For this review, take the finished solid that the model builds, in its own axes (mm). A direction names the side the tool comes from. Round coordinates to 2 decimals unless told otherwise and drop trailing zeros. Loops run counter-clockwise (first coordinate to the right, second up) from the corner with the lowest first, then second, coordinate; pieces in that order, holes last. Notation, with made-up numbers: M 62.5,-7 L 116.5,-7 A19 cw 116.5,11 Z; hole C 67.25,2.25 d2. An arc over 180 degrees is marked long. One line per question, with ' | ' between items. Start each with the question number.
1) We need section C-C (x = -8). Give the boundary of the cut face in (y, z), and give its area (3 significant figures).
2) Mouldability with a two-part tool opening along Z and no side actions: class faces 1 (the face through (-71.05, -17.27, -73.83)), 2 (the face through (-44, 8, -72.784)), 3 (the face through (-44, 15.7, -9)) as pulls with the +Z half, pulls with the -Z half, needs draft (parallel to the pull), parting line crosses it, or undercut.
3) For pin 1 Ø17 at (x, z) = (-32.55, -73.48) entering from -Y; pin 2 Ø6.5 at (x, z) = (-32.55, -73.48) entering from +Y; pin 3 Ø3 at (x, z) = (-74, -68.5) entering from -Y; pin 4 Ø17.5 at (y, z) = (6, -40) entering from -X, all flat-tipped, find the tip position at first contact; note any pin that passes through.
4) For faces 4 (the face through (-44, 21, -49.384)), 5 (the face through (-44, -17, -57.784)), 6 (the face through (-76.39, -6.03, -56.04)), 7 (the face through (-12, 21, -27.09)), list the 3-axis set-ups (+Z, -Z, +X, -X, +Y, -Y) from which the entire face can be reached by the end or side of a thin tool; tool diameter is ignored.
5) For probe 1 along X at (y, z) = (7, -54); probe 2 along X at (y, z) = (17, -56.5); probe 3 along Z at (x, y) = (-67.5, -2.5), list the stretches that pass through material, from the lowest coordinate up. Write a range as from..to.
6) We need section B-B (z = -39). Give the boundary of the cut face in (x, y).
7) We need section A-A (y = -18). State how many separate pieces and enclosed holes the cut face has, and give its area (3 significant figures).
```python
from build123d import *

# Parameters (mm, degrees)
SZKIC1_W                     = 44
SZKIC1_H                     = 78
DODANIE_WYCI_GNI_CIE1_DEPTH  = 15.7
SZKIC2_W                     = 54.82
SZKIC2_H                     = 26
DODANIE_WYCI_GNI_CIE2_DEPTH  = 10
DODANIE_WYCI_GNI_CIE3_DEPTH  = 1
SZKIC6_R                     = 10.4
SZKIC6_R_2                   = 4
DODANIE_WYCI_GNI_CIE4_DEPTH  = 33
SZKIC7_R                     = 10.5
DODANIE_WYCI_GNI_CIE5_DEPTH  = 33
DODANIE_WYCI_GNI_CIE6_DEPTH  = 33
DODANIE_WYCI_GNI_CIE22_DEPTH = 10
SZKIC15_R                    = 3
DODANIE_WYCI_GNI_CIE23_DEPTH = 6.525


with BuildPart() as part:
    # Szkic1 → Dodanie-wyciągnięcie1 (new body)
    with BuildSketch(Plane(origin=(0, 0, 0), x_dir=(1, 0, 0), z_dir=(0, 1, 0))):
        with Locations((-44.05199022, 33.7842123)):
            Rectangle(SZKIC1_W, SZKIC1_H)
    extrude(amount=DODANIE_WYCI_GNI_CIE1_DEPTH)

    # Szkic2 → Dodanie-wyciągnięcie2 (add)
    with BuildSketch(Plane(origin=(0, 15.7, 0), x_dir=(1, 0, 0), z_dir=(0, 1, 0))):
        with Locations((-44.05199022, 36.3842123)):
            Rectangle(SZKIC2_W, SZKIC2_H)
    extrude(amount=DODANIE_WYCI_GNI_CIE2_DEPTH)

    # Szkic3 → Dodanie-wyciągnięcie3 (add)
    with BuildSketch(Plane.XZ):
        with BuildLine():
            Line((-32.55199022, -89.3842123), (-55.55199022, -89.3842123))
            ThreePointArc((-55.55199022, -89.3842123), (-71.45199022, -73.4842123), (-55.55199022, -57.5842123))
            Line((-55.55199022, -57.5842123), (-32.55199022, -57.5842123))
            ThreePointArc((-32.55199022, -57.5842123), (-16.65199022, -73.4842123), (-32.55199022, -89.3842123))
        make_face()
    extrude(amount=DODANIE_WYCI_GNI_CIE3_DEPTH)

    # Szkic6 → Dodanie-wyciągnięcie4 (add)
    with BuildSketch(Plane(origin=(0, -1, 0), x_dir=(-1, 0, 0), z_dir=(0, -1, 0))):
        with Locations((32.55199022, 73.4842123)):
            Circle(SZKIC6_R)
        with Locations((32.55199022, 73.4842123)):
            Circle(SZKIC6_R_2, mode=Mode.SUBTRACT)
        with Locations((55.55199022, 73.4842123)):
            Circle(SZKIC6_R)
        with Locations((55.55199022, 73.4842123)):
            Circle(SZKIC6_R_2, mode=Mode.SUBTRACT)
    extrude(amount=DODANIE_WYCI_GNI_CIE4_DEPTH)

    # Szkic7 → Dodanie-wyciągnięcie5 (add)
    with BuildSketch(Plane(origin=(0, -1, 0), x_dir=(-1, 0, 0), z_dir=(0, -1, 0))):
        with BuildLine():
            Line((55.55199022, 57.9842123), (32.55199022, 57.9842123))
            ThreePointArc((32.55199022, 57.9842123), (17.05199022, 73.4842123), (32.55199022, 88.9842123))
            Line((32.55199022, 88.9842123), (55.55199022, 88.9842123))
            ThreePointArc((55.55199022, 88.9842123), (71.05199022, 73.4842123), (55.55199022, 57.9842123))
        make_face()
        with Locations((55.55199022, 73.4842123)):
            Circle(SZKIC7_R, mode=Mode.SUBTRACT)
        with Locations((32.55199022, 73.4842123)):
            Circle(SZKIC7_R, mode=Mode.SUBTRACT)
    extrude(amount=DODANIE_WYCI_GNI_CIE5_DEPTH)

    # Szkic8 → Dodanie-wyciągnięcie6 (add)
    with BuildSketch(Plane(origin=(0, -1, 0), x_dir=(-1, 0, 0), z_dir=(0, -1, 0))):
        with BuildLine():
            Line((32.55199022, 57.5842123), (55.55199022, 57.5842123))
            ThreePointArc((55.55199022, 57.5842123), (71.45199022, 73.4842123), (55.55199022, 89.3842123))
            Line((55.55199022, 89.3842123), (32.55199022, 89.3842123))
            ThreePointArc((32.55199022, 89.3842123), (16.65199022, 73.4842123), (32.55199022, 57.5842123))
        make_face()
        with BuildLine():
            Line((55.55199022, 57.7842123), (32.55199022, 57.7842123))
            ThreePointArc((32.55199022, 57.7842123), (16.85199022, 73.4842123), (32.55199022, 89.1842123))
            Line((32.55199022, 89.1842123), (55.55199022, 89.1842123))
            ThreePointArc((55.55199022, 89.1842123), (71.25199022, 73.4842123), (55.55199022, 57.7842123))
        make_face(mode=Mode.SUBTRACT)
    extrude(amount=DODANIE_WYCI_GNI_CIE6_DEPTH)

    # Szkic13 → Dodanie-wyciągnięcie22 (add)
    with BuildSketch(Plane(origin=(-16.64199022, 0, 0), x_dir=(0, 0, -1), z_dir=(1, 0, 0))):
        with BuildLine():
            Line((63.214194972, -27.158978782), (48.662895357, 15.7))
            Line((48.662895357, 15.7), (27.090339285, 15.7))
            Line((27.090339285, 15.7), (27.090339285, 25.7))
            Line((27.090339285, 25.7), (59.347416053, 25.7))
            Line((59.347416053, 25.7), (72.7842123, 8.659604885))
            Line((72.7842123, 8.659604885), (77.184359271, 12.129235601))
            Line((77.184359271, 12.129235601), (105.9842123, -20.239479664))
            ThreePointArc((105.9842123, -20.239479664), (86.046845732, -32.647229139), (63.214194972, -27.158978782))
        make_face()
    dodanie_wyci_gni_cie22 = extrude(amount=DODANIE_WYCI_GNI_CIE22_DEPTH)

    # Lustro2: Dodanie-wyciągnięcie22 across plane
    add(dodanie_wyci_gni_cie22.mirror(Plane(origin=(-44.05199022, 0, 0), x_dir=(0, 0, 1), z_dir=(1, 0, 0))))

    # Szkic15 → Dodanie-wyciągnięcie23 (add)
    with BuildSketch(Plane(origin=(-6.64199022, 0, 0), x_dir=(0, 0, -1), z_dir=(1, 0, 0))):
        with Locations((98.903450656, -19.74322341)):
            Circle(SZKIC15_R)
    dodanie_wyci_gni_cie23 = extrude(amount=DODANIE_WYCI_GNI_CIE23_DEPTH)

    # Lustro3: Dodanie-wyciągnięcie23 across plane
    add(dodanie_wyci_gni_cie23.mirror(Plane(origin=(-44.05199022, 0, 0), x_dir=(0, 0, 1), z_dir=(1, 0, 0))))


solid = part.part
```
Answers below:
1) outline: M -27.16,-63.21 A30.42 ccw -20.24,-105.98 L 12.13,-77.18 L 8.66,-72.78 L 25.7,-59.35 L 25.7,-27.09 L 15.7,-27.09 L 15.7,-48.66 Z | area: 2,020 mm^2
2) face 1: undercut | face 2: pulls with the -Z half | face 3: needs draft
3) pin 1: y = -34 | pin 2: y = 15.7 | pin 3: y = -30.91 | pin 4: x = -66.05
4) face 4: -Z, +Y | face 5: -Y | face 6: +Z, -X, -Y | face 7: +Z, +X, +Y, -Y
5) probe 1: -81.46..-71.46, -66.05..-22.05, -16.64..-6.64 | probe 2: -81.46..-71.46, -16.64..-6.64 | probe 3: -83.97..-83.67, -83.36..-63.61, -63.3..-62.99
6) outline: M -81.46,15.7 L -66.05,15.7 L -66.05,0 L -22.05,0 L -22.05,15.7 L -6.64,15.7 L -6.64,25.7 L -81.46,25.7 Z
7) separate pieces: 6 | enclosed holes: 5 | area: 2,320 mm^2
